Here's how the part is built. I have some questions about the finished solid (model axes, mm). A direction names the side the tool comes from. Coordinates: 2 decimals unless noted, no trailing zeros. Order: outer loops, then holes, each group sorted by start corner. A loop starts at its lowest first (then second) coordinate and runs counter-clockwise, first axis right, second up.
```python
from build123d import *

# Parameters (mm, degrees)
F0_W      = 34
F0_H      = 22
F0_R      = 4
F1_DEPTH  = 30.2
F3_DEPTH  = 5
F4_W      = 7.215074
F4_H      = 33.098936
F5_DEPTH  = 40
F7_DEPTH  = 25
F8_R      = 2.5
F9_R      = 3.434689
F10_DEPTH = 40
F14_W     = 3
F14_H     = 33.098936
F15_DEPTH = 40
F16_W     = 12.784926
F16_H     = 2.454489
F17_DEPTH = 40
F19_DEPTH = 25


with BuildPart() as f1:
    # F0 (on Front) → F1 (new body)
    with BuildSketch(Plane.XZ):
        with Locations((-19.066667, -4.857694)):
            Rectangle(F0_W, F0_H)
        with Locations((-19.066667, -4.857694)):
            Circle(F0_R, mode=Mode.SUBTRACT)
        with Locations((17.733333, -4.857694)):
            Rectangle(F0_W, F0_H)
        with Locations((17.733333, -4.857694)):
            Circle(F0_R, mode=Mode.SUBTRACT)
    extrude(amount=F1_DEPTH)


with BuildPart() as f3:
    # F2 (on face) → F3 (new body)
    with BuildSketch(Plane.XY.offset(6.142306)):
        Polygon((-2.548193, 1.449468), (-40.917817, 1.449468), (-40.917817, -31.649468), (35.821432, -31.649468), (35.821432, 1.449468), align=None)
        with BuildLine():
            Line((-30.548193, -24.5), (-33.048193, -24.5))
            ThreePointArc((-33.048193, -24.5), (-35.548193, -22), (-33.048193, -19.5))
            Line((-33.048193, -19.5), (-30.548193, -19.5))
            ThreePointArc((-30.548193, -19.5), (-28.048193, -22), (-30.548193, -24.5))
        make_face(mode=Mode.SUBTRACT)
        with BuildLine():
            ThreePointArc((27.951807, -19.5), (30.451807, -22), (27.951807, -24.5))
            Line((27.951807, -24.5), (25.451807, -24.5))
            ThreePointArc((25.451807, -24.5), (22.951807, -22), (25.451807, -19.5))
            Line((25.451807, -19.5), (27.951807, -19.5))
        make_face(mode=Mode.SUBTRACT)
        with BuildLine():
            Line((-30.548193, -6.5), (-33.048193, -6.5))
            ThreePointArc((-33.048193, -6.5), (-35.548193, -4), (-33.048193, -1.5))
            Line((-33.048193, -1.5), (-30.548193, -1.5))
            ThreePointArc((-30.548193, -1.5), (-28.048193, -4), (-30.548193, -6.5))
        make_face(mode=Mode.SUBTRACT)
        with BuildLine():
            Line((25.451807, -1.5), (27.951807, -1.5))
            ThreePointArc((27.951807, -1.5), (30.451807, -4), (27.951807, -6.5))
            Line((27.951807, -6.5), (25.451807, -6.5))
            ThreePointArc((25.451807, -6.5), (22.951807, -4), (25.451807, -1.5))
        make_face(mode=Mode.SUBTRACT)
    extrude(amount=F3_DEPTH)

    # F4 (on face) → F5 (join)
    with BuildSketch(Plane.XY.offset(11.142306)):
        with Locations((19.428969, -15.1)):
            Rectangle(F4_W, F4_H)
    extrude(amount=F5_DEPTH)

    # F6 (on face) → F7 (cut)
    with BuildSketch(Plane(origin=(15.821432, 0, 0), x_dir=(0, -1, 0), z_dir=(-1, 0, 0))):
        with BuildLine():
            ThreePointArc((15.1, 33.392306), (16.337437, 33.904869), (16.85, 35.142306))
            ThreePointArc((16.85, 35.142306), (13.862563, 36.379742), (15.1, 33.392306))
        make_face()
    extrude(amount=-F7_DEPTH, mode=Mode.SUBTRACT)

    # F8
    f8_edges = [f3.edges().sort_by_distance(p)[0] for p in [
        (19.428969, 1.449468, 51.142306),
        (19.428969, -31.649468, 51.142306),
    ]]
    fillet(f8_edges, radius=F8_R)

    # F9 (on face) → F10 (cut, through all)
    with BuildSketch(Plane.XY.offset(51.142306)):
        with Locations((25.451807, -4)):
            Circle(F9_R)
        with Locations((25.451807, -22)):
            Circle(F9_R)
    extrude(amount=-F10_DEPTH, mode=Mode.SUBTRACT)

    # F14 (on face) → F15 (cut, through all)
    with BuildSketch(Plane.XY.offset(51.142306)):
        with Locations((17.321432, -15.1)):
            Rectangle(F14_W, F14_H)
    extrude(amount=-F15_DEPTH, mode=Mode.SUBTRACT)

    # F16 (on face) → F17 (join, through all)
    with BuildSketch(Plane.XY.offset(11.142306)):
        with Locations((29.428969, -9.451033)):
            Rectangle(F16_W, F16_H)
    extrude(amount=F17_DEPTH)

    # F18 (on face) → F19 (cut)
    with BuildSketch(Plane.XZ.offset(10.678278)):
        Polygon((35.821432, 51.142306), (23.036506, 51.142306), (35.821432, 11.142306), align=None)
    extrude(amount=-F19_DEPTH, mode=Mode.SUBTRACT)


with BuildPart() as f11_1:
    # F11: copy of F3
    add(f3.part)


solid = f3.part
```
Q1. If we section it at B-B on y = -4: Write out the boundary of the cut face in (x, z), then the cut area to 3 significant figures.
Q2. If we section it at D-D on x = 4.5: Write out the boundary of the cut face in (y, z), then the cut area to 3 significant figures.
Q3. We'd pull the mould along X, two halves only. Please class faces 1 (the cylindrical face through (30.45, -21.95, 8.61)), 2 (the cylindrical face through (-28.05, -3.95, 8.61)), 3 (the flat face through (23.037, -28, 31)), 4 (the flat face through (30, -2, 11.142)): pulls with the +X half, pulls with the -X half, needs draft (parallel to the pull), parting line crosses it, or undercut.
Q4. If we section it at C-C on z = 18: Write out the boundary of the cut face in (x, y), then the cut area to 3 significant figures.
Q5. If we section it at A-A on z = 10: Write out the boundary of the cut face in (x, y).
Q6. Will these pins go through, and if not, where does the flat tip stop? pin 1 (4.5 mm diameter, centred on y = -13.5, z = 32, fed in from +X); pin 2 (10 mm diameter, centred on x = -20.5, y = -8, fed in from +Z); pin 3 (10 mm diameter, centred on x = 30.5, z = 35.5, fed in from +Y).
Q7. For faces 5 (the flat face through (28, -10.678, 26)), 6 (the flat face through (23.037, -7, 31)), 7 (the flat face through (-11, -15, 11.142)), 8 (the flat face through (-32, -6.5, 9)), which set-ups out of +Z, -Z, +X, -X, +Y, -Y let a thin tool reach every point of the face, with its end or its side?
Q8. I need wall thicknesses on L1, parallel to Z at x = 21.8, y = -15.1; L2, parallel to X at y = -29, z = 37.5; L3, parallel to Y at x = 33, z = 19. Which ranges of each line are inside material? Lowest first, please.
Reply:
1. outline: (-40.92, 6.14) - (-35.55, 6.14) - (-35.55, 11.14) - (-40.92, 11.14) - close; (-28.05, 6.14) - (22.95, 6.14) - (22.95, 11.14) - (22.02, 11.14) - (22.02, 51.14) - (18.82, 51.14) - (18.82, 11.14) - (-28.05, 11.14) - close; (30.45, 6.14) - (35.82, 6.14) - (35.82, 11.14) - (30.45, 11.14) - close
1. area: 437 mm2
2. outline: (-31.65, 6.14) - (1.45, 6.14) - (1.45, 11.14) - (-31.65, 11.14) - close
2. area: 165 mm2
3. face 1: undercut
3. face 2: undercut
3. face 3: pulls with the +X half
3. face 4: needs draft
4. outline: (18.82, -31.65) - (23.04, -31.65) - (23.04, -24.44) arc R3.43 cw to (23.04, -19.56) - (23.04, -10.68) - (33.63, -10.68) - (33.63, -8.22) - (23.04, -8.22) - (23.04, -6.44) arc R3.43 cw to (23.04, -1.56) - (23.04, 1.45) - (18.82, 1.45) - close
4. area: 159 mm2
5. outline: (-40.92, -31.65) - (35.82, -31.65) - (35.82, 1.45) - (-40.92, 1.45) - close; hole (-33.05, -24.5) - (-30.55, -24.5) arc R2.5 ccw to (-30.55, -19.5) - (-33.05, -19.5) arc R2.5 ccw to start; hole (-33.05, -6.5) - (-30.55, -6.5) arc R2.5 ccw to (-30.55, -1.5) - (-33.05, -1.5) arc R2.5 ccw to start; hole (25.45, -24.5) - (27.95, -24.5) arc R2.5 ccw to (27.95, -19.5) - (25.45, -19.5) arc R2.5 ccw to start; hole (25.45, -6.5) - (27.95, -6.5) arc R2.5 ccw to (27.95, -1.5) - (25.45, -1.5) arc R2.5 ccw to start
6. pin 1: stops at x = 23.04
6. pin 2: stops at z = 11.14
6. pin 3: stops at y = -8.22
7. face 5: +Z, +X, -Y
7. face 6: +Z, +X, +Y
7. face 7: +Z, -X, +Y, -Y
7. face 8: +Z, -Z
8. L1: z = 6.14 to 33.39, 36.89 to 51.14
8. L2: x = 18.82 to 23.04
8. L3: y = -10.68 to -8.22
